Here's how the part is built. I have some questions about the finished solid (model axes, mm). A direction names the side the tool comes from. Coordinates: 2 decimals unless noted, no trailing zeros. Write each loop counter-clockwise with the first axis right and the second up, starting at its lowest first coordinate (ties: lowest second). Pieces come first, ordered by that corner, then holes. Notation, with made-up numbers: (21, 74) -> (57, 74) arc R26 ccw to (57, 105) -> close; hole circle Ø9 at (60.5, 35.5). An arc over 180 degrees is marked (long way). Put each result on its own line as item: value.
```python
from build123d import *

# Parameters (mm, degrees)
F0_W     = 60
F0_H     = 60
F1_DEPTH = 60
F2_W     = 30
F2_H     = 30


with BuildPart() as f1:
    # F0 (on Front) → F1 (new body)
    with BuildSketch(Plane.XZ):
        with Locations((-30, -30)):
            Rectangle(F0_W, F0_H)
    extrude(amount=F1_DEPTH)

    # F2 (on face) → F3 (revolve)
    with BuildSketch(Plane(origin=(0, 0, 0), x_dir=(-1, 0, 0), z_dir=(0, 1, 0))):
        with Locations((-15, -27.4707084894)):
            Rectangle(F2_W, F2_H)
        Polygon((0, -12.4707084894), (0, -42.4707084894), (0, -60), (60, -60), (60, 0), (0, 0), align=None)
    revolve(axis=Axis((0, 0, -27.4707084894), (0, 0, 1)))


solid = f1.part
```
Item 1: For P1, Ø6, axis at y = 47, z = -49.5, coming from the -X side; P2, Ø5, axis at x = -13, z = -9.5, coming from the +Y side; P3, Ø1.5, axis at y = 15, z = -29, coming from the +X side, each with a flat end and sliding along its axis, tell me the tip position at first contact or that it passes through.
Output:
P1: stops at x = -40.79
P2: stops at y = 59.07
P3: stops at x = 58.28
Item 2: Please list where these lines run through material, in increasing order: line 1 along Z through (x, y) = (0, 12.5); line 2 along Y through (x, z) = (24, -31); line 3 along Y through (x, z) = (-2, -30). Write a range as from..to.
Output:
line 1: z = -60..-42.47, -12.47..0
line 2: y = -54.99..-18, 18..54.99
line 3: y = -60..0, 29.93..59.97
Item 3: Imagine slicing it at D-D on z = -47. Write out the boundary of the cut face in (x, y), then the cut area to 3 significant figures.
Output:
outline: (-60, -60) -> (0, -60) arc R60 ccw (long way) to (-60, 0) -> close
area: 12,100 mm²
Item 4: Imagine slicing it at B-B on y = 7. Write out the boundary of the cut face in (x, z), then the cut area to 3 significant figures.
Output:
outline: (-59.59, -60) -> (59.59, -60) -> (59.59, 0) -> (-59.59, 0) -> close; hole (-29.17, -42.47) -> (29.17, -42.47) -> (29.17, -12.47) -> (-29.17, -12.47) -> close
area: 5,400 mm²
Item 5: If we mould it in two halves opening along Z, with no side actions, what happens to faces 3 (the flat face through (-15, 0, -27)), 4 (the cylindrical face through (43.803, 41.004, -29.58)), 5 (the flat face through (6, 7, -12.471)), 6 (the flat face through (-1, -1, -60))? For each: released by +Z, released by -Z, zero draft, split by the parting line, or undercut.
Output:
face 3: undercut
face 4: zero draft
face 5: undercut
face 6: released by -Z
Item 6: Imagine slicing it at A-A on z = -32. Write out the boundary of the cut face in (x, y), then the cut area to 3 significant figures.
Output:
outline: (-60, -60) -> (0, -60) arc R60 ccw (long way) to (-60, 0) -> close; hole (-30, 0) -> (0, 0) -> (0, -30) arc R30 ccw (long way) to start
area: 9,960 mm²
Item 7: Imagine slicing it at C-C on x = 20. Write out the boundary of the cut face in (y, z), then the cut area to 3 significant figures.
Output:
outline: (-56.57, -60) -> (56.57, -60) -> (56.57, 0) -> (-56.57, 0) -> close; hole (-22.36, -42.47) -> (22.36, -42.47) -> (22.36, -12.47) -> (-22.36, -12.47) -> close
area: 5,450 mm²
Item 8: Which directions (+Z, -Z, +X, -X, +Y, -Y) give clear straight access to the entire face, cutting with the end or side of a thin tool? Please do faces 1 (the flat face through (6, 7, -42.471)), 2 (the flat face through (-30, -60, -30)).
Output:
face 1: none
face 2: +Z, -Z, +X, -X, -Y
